Design review of the part built by this model. Coordinates are the model's own, in mm. Face numbers are marked on the shaded views. A direction names the side the tool comes from. Round coordinates to 2 decimals unless told otherwise and drop trailing zeros. Loops run counter-clockwise (first coordinate to the right, second up) from the corner with the lowest first, then second, coordinate; pieces in that order, holes last. Notation, with made-up numbers: (18, 62) -> (36, 62) arc R24 ccw to (36, 98) -> close; hole circle Ø8 at (-28, 60.5). An arc over 180 degrees is marked (long way). Use a Markdown table: item, result. Add a question column.
from build123d import *

# Parameters (mm, degrees)
BASE_FLANGE1_DEPTH             = 700
CUT_EXTRUDE1_REACH             = 704.282
CUT_EXTRUDE1_DIRECTION_2_REACH = 704.282


# Sheet-metal steps are written as plain solids
with BuildPart() as part:
    # Sketch1 → Base-Flange1 (new body)
    with BuildSketch(Plane(origin=(0, 0, 0), x_dir=(1, 0, 0), z_dir=(0, 1, 0))):
        with BuildLine():
            Line((-40, -40), (-40, -3.7366))
            ThreePointArc((-40, -3.7366), (-38.905575199, -1.094424801), (-36.2634, 0))
            Line((-36.2634, 0), (36.2634, 0))
            ThreePointArc((36.2634, 0), (38.905575199, -1.094424801), (40, -3.7366))
            Line((40, -3.7366), (40, -40))
            Line((40, -40), (37, -40))
            Line((37, -40), (37, -3.7366))
            ThreePointArc((37, -3.7366), (36.784254855, -3.215745145), (36.2634, -3))
            Line((36.2634, -3), (-36.2634, -3))
            ThreePointArc((-36.2634, -3), (-36.784254855, -3.215745145), (-37, -3.7366))
            Line((-37, -3.7366), (-37, -40))
            Line((-37, -40), (-40, -40))
        make_face()
    extrude(amount=BASE_FLANGE1_DEPTH)

    # Cut-Extrude1: up to this face of the body (flat: up to its plane)
    cut_extrude1_end = Plane(part.part.faces().sort_by_distance((-40, 350, 21.8683))[0])
    # Sketch6 → Cut-Extrude1 (cut, up to the picked face)
    with BuildSketch(Plane(origin=(0, 0, 0), x_dir=(0, 0, -1), z_dir=(1, 0, 0)), mode=Mode.PRIVATE) as cut_extrude1_sk1:
        Polygon((-8.7366, 700), (-40, 630), (-40, 700), align=None)
    cut_extrude1_tool1 = split(extrude(cut_extrude1_sk1.sketch, amount=-CUT_EXTRUDE1_REACH, mode=Mode.PRIVATE), bisect_by=cut_extrude1_end, keep=Keep.BOTH, mode=Mode.PRIVATE)
    add(cut_extrude1_tool1.solids().sort_by(Axis((0, 676.666667, 29.578867), (-1, 0, 0)))[0], mode=Mode.SUBTRACT)

    # Cut-Extrude1 direction 2: up to this face of the body (flat: up to its plane)
    cut_extrude1_direction_2_end = Plane(part.part.faces().sort_by_distance((40, 350, 21.8683))[0])
    # Sketch6 → Cut-Extrude1 direction 2 (cut, up to the picked face)
    with BuildSketch(Plane(origin=(0, 0, 0), x_dir=(0, 0, -1), z_dir=(1, 0, 0)), mode=Mode.PRIVATE) as cut_extrude1_direction_2_sk1:
        Polygon((-8.7366, 700), (-40, 630), (-40, 700), align=None)
    cut_extrude1_direction_2_tool1 = split(extrude(cut_extrude1_direction_2_sk1.sketch, amount=CUT_EXTRUDE1_DIRECTION_2_REACH, mode=Mode.PRIVATE), bisect_by=cut_extrude1_direction_2_end, keep=Keep.BOTH, mode=Mode.PRIVATE)
    add(cut_extrude1_direction_2_tool1.solids().sort_by(Axis((0, 676.666667, 29.578867), (1, 0, 0)))[0], mode=Mode.SUBTRACT)


solid = part.part
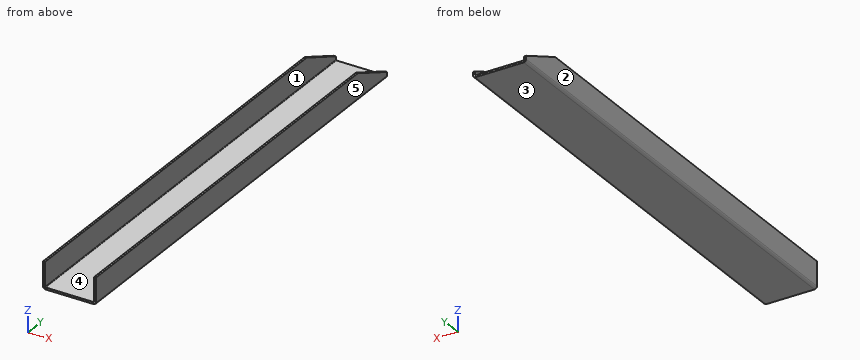
1. Consider section C-C on x = -2. State the section outline as (y, z) points.
2. For the marked faces 1 and 2, list the 3-axis set-ups (+Z, -Z, +X, -X, +Y, -Y) from which the entire face can be reached by the end or side of a thin tool; tool diameter is ignored.
3. Mouldability with a two-part tool opening along X and no side actions: class the marked faces 3, 4 and 5 as +X half, -X half, draft (parallel to the pull), parting line (faces both ways), or undercut.
4. Consider section B-B on y = 117.5. State the section outline as (x, z) points.
5. To check wall thickness, follow probe 1 along X at (y, z) = (196.5, 26.5); probe 2 along Z at (x, y) = (-20, 266). State the ranges of each line that lie inside material, in increasing order. Write a range as from..to.
6. Consider section A-A on z = 31.5. State the section outline as (x, y) points.
Verdict:
| question | item | result |
|---|---|---|
| 1 | outline | (0, 0) -> (700, 0) -> (700, 3) -> (0, 3) -> close |
| 2 | face 1 | +Z, +Y, -Y |
| 2 | face 2 | +Z, -Z, -X, +Y, -Y |
| 3 | face 3 | draft |
| 3 | face 4 | undercut |
| 3 | face 5 | +X half |
| 4 | outline | (-40, 3.74) arc R3.74 ccw to (-36.26, 0) -> (36.26, 0) arc R3.74 ccw to (40, 3.74) -> (40, 40) -> (37, 40) -> (37, 3.74) arc R0.74 cw to (36.26, 3) -> (-36.26, 3) arc R0.74 cw to (-37, 3.74) -> (-37, 40) -> (-40, 40) -> close |
| 5 | probe 1 | x = -40..-37, 37..40 |
| 5 | probe 2 | z = 0..3 |
| 6 | outline | (-40, 0) -> (-37, 0) -> (-37, 649.03) -> (-40, 649.03) -> close; (37, 0) -> (40, 0) -> (40, 649.03) -> (37, 649.03) -> close |
